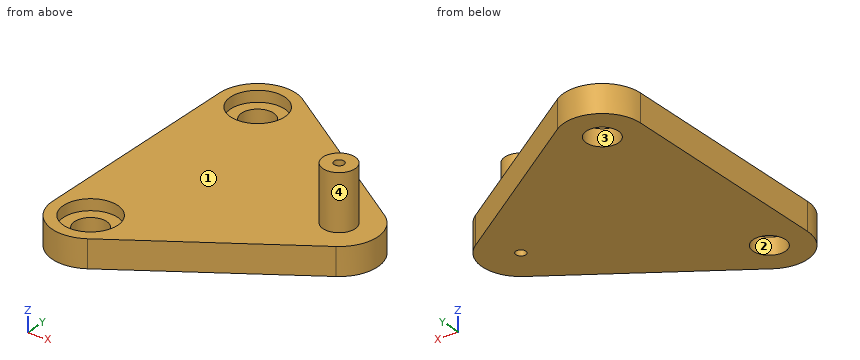
from build123d import *

# Parameters (mm, degrees)
CROQUIS1_R              = 1.45
SALIENTE_EXTRUIR1_DEPTH = 2.5
CROQUIS2_R              = 2.45
CORTAR_EXTRUIR1_DEPTH   = 1
CROQUIS3_R              = 1.45
CROQUIS3_R_2            = 0.45
SALIENTE_EXTRUIR2_DEPTH = 5
CROQUIS4_R              = 0.45
CORTAR_EXTRUIR2_DEPTH   = 24.392907579


with BuildPart() as part:
    # Croquis1 → Saliente-Extruir1 (new body)
    with BuildSketch(Plane.XY):
        with BuildLine():
            Line((-3.45, 10), (-3.45, -10))
            ThreePointArc((-3.45, -10), (-1.630018545, -13.040647882), (1.909733068, -12.873224601))
            Line((1.909733068, -12.873224601), (16.923571713, -2.89404507))
            ThreePointArc((16.923571713, -2.89404507), (18.475, 0), (16.923571713, 2.89404507))
            Line((16.923571713, 2.89404507), (1.909733068, 12.873224601))
            ThreePointArc((1.909733068, 12.873224601), (-1.630018545, 13.040647882), (-3.45, 10))
        make_face()
        with Locations((0, 10)):
            Circle(CROQUIS1_R, mode=Mode.SUBTRACT)
        with Locations(Location((0, -10, 0), (0, 0, 180))):
            Circle(CROQUIS1_R, mode=Mode.SUBTRACT)
    extrude(amount=SALIENTE_EXTRUIR1_DEPTH)

    # Croquis2 → Cortar-Extruir1 (cut)
    with BuildSketch(Plane.XY.offset(2.5)):
        with Locations((0, 10)):
            Circle(CROQUIS2_R)
        with Locations((0, -10)):
            Circle(CROQUIS2_R)
    extrude(amount=-CORTAR_EXTRUIR1_DEPTH, mode=Mode.SUBTRACT)

    # Croquis3 → Saliente-Extruir2 (add)
    with BuildSketch(Plane.XY.offset(2.5)):
        with Locations((15, 0)):
            Circle(CROQUIS3_R)
        with Locations((15, 0)):
            Circle(CROQUIS3_R_2, mode=Mode.SUBTRACT)
    extrude(amount=SALIENTE_EXTRUIR2_DEPTH)

    # Croquis4 → Cortar-Extruir2 (cut, through all)
    with BuildSketch(Plane.XY.offset(2.5)):
        with Locations((15, 0)):
            Circle(CROQUIS4_R)
    extrude(amount=-CORTAR_EXTRUIR2_DEPTH, mode=Mode.SUBTRACT)


solid = part.part
For this review, take the finished solid that the model builds, in its own axes (mm). Face numbers are marked on the shaded views. Give positions to 0.01 mm unless a question says otherwise; leave off trailing zeros. Loops run counter-clockwise (first coordinate to the right, second up) from the corner with the lowest first, then second, coordinate; pieces in that order, holes last.
Item 1: Take a section at D-D, the plane z = 3.75. State the section outline as (x, y) points.
Item 2: Insertion check: pin 1 (4 mm diameter, centred on x = -1, y = 9.5, fed in from +Z); pin 2 (2.5 mm diameter, centred on x = 0.5, y = -11, fed in from +Z); pin 3 (2 mm diameter, centred on x = 16, z = 6, fed in from -Y). Each pin has a flat end and moves straight along its axis. Give the tip position at first contact, or say it passes through.
Item 3: Take a section at C-C, the plane x = 15. State the section outline as (y, z) points.
Item 4: Take a section at B-B, the plane x = 0. State the section outline as (y, z) points, and give its area (4 significant figures).
Item 5: Draft analysis for pull direction Y (two halves, no side actions). For the marked faces 1, 2, 3 and 4, state which applies: +Y half, -Y half, draft (parallel to the pull), parting line (faces both ways), or undercut.
Item 6: For line 1 along Y through (x, z) = (0, 1.85); line 2 along Y through (x, z) = (0, 0.95); line 3 along Y through (x, z) = (15, 5.1), list the stretches that pass through material, from the lowest coordinate up.
Item 7: Take a section at A-A, the plane y = 0. State the section outline as (x, z) points (3 decimals), and give its area (3 significant figures).
Calculated:
1. outline: circle Ø2.9 at (15, 0); hole circle Ø0.9 at (15, 0)
2. pin 1: stops at z = 2.5
2. pin 2: stops at z = 1.5
2. pin 3: stops at y = -1.45
3. outline: (-4.17, 0) - (-0.45, 0) - (-0.45, 7.5) - (-1.45, 7.5) - (-1.45, 2.5) - (-4.17, 2.5) - close; (0.45, 0) - (4.17, 0) - (4.17, 2.5) - (1.45, 2.5) - (1.45, 7.5) - (0.45, 7.5) - close
4. outline: (-13.45, 0) - (-11.45, 0) - (-11.45, 1.5) - (-12.45, 1.5) - (-12.45, 2.5) - (-13.45, 2.5) - close; (-8.55, 0) - (8.55, 0) - (8.55, 1.5) - (7.55, 1.5) - (7.55, 2.5) - (-7.55, 2.5) - (-7.55, 1.5) - (-8.55, 1.5) - close; (11.45, 0) - (13.45, 0) - (13.45, 2.5) - (12.45, 2.5) - (12.45, 1.5) - (11.45, 1.5) - close
4. area: 48.75 mm2
5. face 1: draft
5. face 2: undercut
5. face 3: undercut
5. face 4: parting line
6. line 1: y = -13.45 to -12.45, -7.55 to 7.55, 12.45 to 13.45
6. line 2: y = -13.45 to -11.45, -8.55 to 8.55, 11.45 to 13.45
6. line 3: y = -1.45 to -0.45, 0.45 to 1.45
7. outline: (-3.45, 0) - (14.55, 0) - (14.55, 7.5) - (13.55, 7.5) - (13.55, 2.5) - (-3.45, 2.5) - close; (15.45, 0) - (18.475, 0) - (18.475, 2.5) - (16.45, 2.5) - (16.45, 7.5) - (15.45, 7.5) - close
7. area: 62.6 mm2
